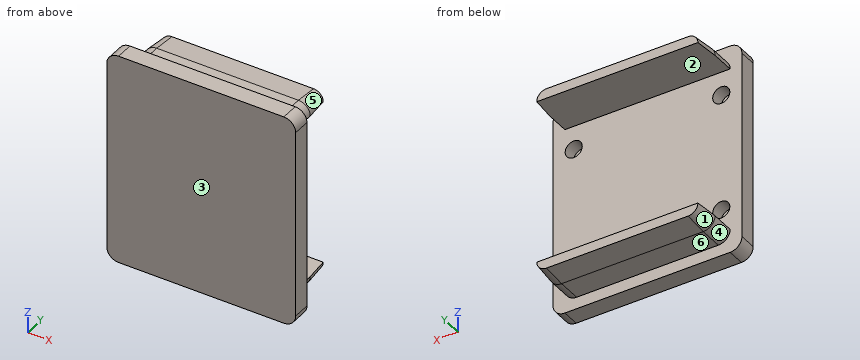
```python
from build123d import *
from OCP.BRepFilletAPI import BRepFilletAPI_MakeChamfer

# Parameters (mm, degrees)
SKETCH1_W                                  = 32
SKETCH1_H                                  = 36
BOSS_EXTRUDE1_DEPTH                        = 3
SKETCH4_W                                  = 28
SKETCH4_H                                  = 2
BOSS_EXTRUDE3_DEPTH                        = 8
FILLET4_R                                  = 2
CHAMFER2_SIZE                              = 4
CHAMFER2_SIZE2                             = 0.349954654
SKETCH5_R                                  = 1.45
CUT_EXTRUDE1_DEPTH                         = 2.3
MIRROR1_AT_THE_SECOND_PLANE_COPY_1_SKETC_R = 1.45
MIRROR1_AT_THE_SECOND_PLANE_COPY_1_DEPTH   = 2.3


with BuildPart() as part:
    # Sketch1 → Boss-Extrude1 (new body)
    with BuildSketch(Plane(origin=(0, 0, 0), x_dir=(1, 0, 0), z_dir=(0, 1, 0))):
        Rectangle(SKETCH1_W, SKETCH1_H)
    extrude(amount=BOSS_EXTRUDE1_DEPTH)

    # Sketch4 → Boss-Extrude3 (add)
    with BuildSketch(Plane(origin=(0, 3, 0), x_dir=(1, 0, 0), z_dir=(0, 1, 0))):
        with Locations((0, 15)):
            Rectangle(SKETCH4_W, SKETCH4_H)
        with Locations((0, -15)):
            Rectangle(SKETCH4_W, SKETCH4_H)
    extrude(amount=BOSS_EXTRUDE3_DEPTH)

    # Fillet4
    fillet4_edges = [part.edges().sort_by_distance(p)[0] for p in [
        (14, 7, -16),
        (14, 7, 16),
        (-16, 1.5, 18),
        (16, 1.5, 18),
        (-16, 1.5, -18),
        (16, 1.5, -18),
        (-14, 7, 16),
        (-14, 7, -16),
    ]]
    fillet(fillet4_edges, radius=FILLET4_R - 0.0001)  # a hair under: the kernel refuses the full size

    # Chamfer2: one chamfer whose edges measure the first distance from different faces: ONE call of the kernel's chamfer builder (chamfer() names one face for all edges)
    chamfer2_edges_1 = [part.edges().sort_by_distance(p)[0] for p in [
        (0, 11, 16),
    ]]
    chamfer2_side_1 = [part.faces().sort_by_distance(p)[0] for p in [
        (0, 7, 16),
    ]]
    chamfer2_edges_2 = [part.edges().sort_by_distance(p)[0] for p in [
        (13.414242852, 11, 15.414242852),
    ]]
    chamfer2_side_2 = [part.faces().sort_by_distance(p)[0] for p in [
        (13.414242852, 7, 15.414242852),
    ]]
    chamfer2_edges_3 = [part.edges().sort_by_distance(p)[0] for p in [
        (-13.414242852, 11, 15.414242852),
    ]]
    chamfer2_side_3 = [part.faces().sort_by_distance(p)[0] for p in [
        (-13.414242852, 7, 15.414242852),
    ]]
    chamfer2_edges_4 = [part.edges().sort_by_distance(p)[0] for p in [
        (0, 11, -16),
    ]]
    chamfer2_side_4 = [part.faces().sort_by_distance(p)[0] for p in [
        (0, 7, -16),
    ]]
    chamfer2_edges_5 = [part.edges().sort_by_distance(p)[0] for p in [
        (13.414242852, 11, -15.414242852),
    ]]
    chamfer2_side_5 = [part.faces().sort_by_distance(p)[0] for p in [
        (13.414242852, 7, -15.414242852),
    ]]
    chamfer2_edges_6 = [part.edges().sort_by_distance(p)[0] for p in [
        (-13.414242852, 11, -15.414242852),
    ]]
    chamfer2_side_6 = [part.faces().sort_by_distance(p)[0] for p in [
        (-13.414242852, 7, -15.414242852),
    ]]
    chamfer2 = BRepFilletAPI_MakeChamfer(part.part.solid().wrapped)
    for e in chamfer2_edges_1:
        chamfer2.Add(CHAMFER2_SIZE, CHAMFER2_SIZE2, e.wrapped, chamfer2_side_1[0].wrapped)  # the first distance lies on this face
    for e in chamfer2_edges_2:
        chamfer2.Add(CHAMFER2_SIZE, CHAMFER2_SIZE2, e.wrapped, chamfer2_side_2[0].wrapped)  # the first distance lies on this face
    for e in chamfer2_edges_3:
        chamfer2.Add(CHAMFER2_SIZE, CHAMFER2_SIZE2, e.wrapped, chamfer2_side_3[0].wrapped)  # the first distance lies on this face
    for e in chamfer2_edges_4:
        chamfer2.Add(CHAMFER2_SIZE, CHAMFER2_SIZE2, e.wrapped, chamfer2_side_4[0].wrapped)  # the first distance lies on this face
    for e in chamfer2_edges_5:
        chamfer2.Add(CHAMFER2_SIZE, CHAMFER2_SIZE2, e.wrapped, chamfer2_side_5[0].wrapped)  # the first distance lies on this face
    for e in chamfer2_edges_6:
        chamfer2.Add(CHAMFER2_SIZE, CHAMFER2_SIZE2, e.wrapped, chamfer2_side_6[0].wrapped)  # the first distance lies on this face
    add(Compound.cast(chamfer2.Shape()), mode=Mode.REPLACE)

    # Sketch5 → Cut-Extrude1 (cut)
    with BuildSketch(Plane(origin=(0, 3, 0), x_dir=(1, 0, 0), z_dir=(0, 1, 0))):
        with Locations(Location((-12.5, 10, 0), (0, 0, 270))):
            Circle(SKETCH5_R)
    cut_extrude1 = extrude(amount=-CUT_EXTRUDE1_DEPTH, mode=Mode.SUBTRACT)

    # Mirror1: Cut-Extrude1 across plane
    add(cut_extrude1.mirror(Plane(origin=(0, 0, 0), x_dir=(0, 0, 1), z_dir=(1, 0, 0))), mode=Mode.SUBTRACT)

    # Mirror1 at the second plane: Cut-Extrude1 across plane
    add(cut_extrude1.mirror(Plane.XY), mode=Mode.SUBTRACT)

    # Mirror1 at the second plane copy 1 sketc → Mirror1 at the second plane copy 1 (cut)
    with BuildSketch(Plane(origin=(0, 3, 0), x_dir=(-1, 0, 0), z_dir=(0, 1, 0))):
        with Locations(Location((-12.5, 10, 0), (0, 0, 270))):
            Circle(MIRROR1_AT_THE_SECOND_PLANE_COPY_1_SKETC_R)
    extrude(amount=-MIRROR1_AT_THE_SECOND_PLANE_COPY_1_DEPTH, mode=Mode.SUBTRACT)


solid = part.part
```
Source: CAD feature listing. Evaluate the final solid. Frame: model axes, mm. Face numbers are marked on the shaded views. A direction names the side the tool comes from. Round coordinates to 2 decimals unless told otherwise and drop trailing zeros. Order: outer loops, then holes, each group sorted by start corner. A loop starts at its lowest first (then second) coordinate and runs counter-clockwise, first axis right, second up. Notation, with made-up numbers: (8, 11) -> (66, 11) arc R10 cw to (66, 25) -> close; hole circle Ø4 at (9, -17.5). An arc over 180 degrees is marked (long way). One line per item, written item: value. Start each with the question number.
Q1. Section query A-A (y = 2). Return the cut outline in (x, z).
Q2. Draft query along Z for the marked faces 1, 2 and 3. Return one class per face: pulls with the +Z half, pulls with the -Z half, needs draft (parallel to the pull), parting line crosses it, or undercut.
Q3. Section query D-D (z = -10). Return the cut outline in (x, y), plus the area to 3 significant figures.
Q4. Material intervals for probe 1 along Z at (x, y) = (12.5, 1.9); probe 2 along X at (y, z) = (1.5, -10); probe 3 along Z at (x, y) = (-9.5, 6.75), sorted ascending.
Q5. Pin query (flat end, axial travel): pin 1 (1.7 mm diameter, centred on x = -12.5, z = 10, fed in from +Y); pin 2 (5 mm diameter, centred on x = -12, z = -3, fed in from +Y); pin 3 (5 mm diameter, centred on x = -7, z = 13.5, fed in from -Y); pin 4 (2 mm diameter, centred on x = 9, y = 7.5, fed in from -Z). Return the tip coordinate at first contact, or that it passes through.
Q6. Section query B-B (x = 2.5). Return the cut outline in (y, z), plus the area to 3 significant figures.
Q7. Access query for the marked faces 4, 5 and 6. Directions: +Z, -Z, +X, -X, +Y, -Y. A direction counts if a zero-diameter tool reaches every point of the face in a straight line with its end or side. Return the directions, or none.
Findings below:
1. outline: (-16, -16) arc R2 ccw to (-14, -18) -> (14, -18) arc R2 ccw to (16, -16) -> (16, 16) arc R2 ccw to (14, 18) -> (-14, 18) arc R2 ccw to (-16, 16) -> close; hole circle Ø2.9 at (-12.5, -10); hole circle Ø2.9 at (-12.5, 10); hole circle Ø2.9 at (12.5, -10); hole circle Ø2.9 at (12.5, 10)
2. face 1: pulls with the -Z half
2. face 2: undercut
2. face 3: needs draft
3. outline: (-16, 0) -> (16, 0) -> (16, 3) -> (13.95, 3) -> (13.95, 0.7) -> (11.05, 0.7) -> (11.05, 3) -> (-11.05, 3) -> (-11.05, 0.7) -> (-13.95, 0.7) -> (-13.95, 3) -> (-16, 3) -> close
3. area: 82.7 mm²
4. probe 1: -18 to -11.45, -8.55 to 8.55, 11.45 to 18
4. probe 2: -16 to -13.95, -11.05 to 11.05, 13.95 to 16
4. probe 3: -16 to -14, 14 to 16
5. pin 1: y = 0.7
5. pin 2: y = 3
5. pin 3: y = 0
5. pin 4: z = -16
6. outline: (0, -18) -> (3, -18) -> (3, -16) -> (7, -16) -> (11, -15.65) -> (11, -14) -> (3, -14) -> (3, 14) -> (11, 14) -> (11, 15.65) -> (7, 16) -> (3, 16) -> (3, 18) -> (0, 18) -> close
6. area: 139 mm²
7. face 4: -Z, -X, +Y
7. face 5: +Z, +X, +Y
7. face 6: -Z, +X, -X, +Y
